Read the model definition and answer for the solid it produces. Units are mm, in the model's axes. A direction names the side the tool comes from. Coordinates: 2 decimals unless noted, no trailing zeros. Loops run counter-clockwise (first coordinate to the right, second up) from the corner with the lowest first, then second, coordinate; pieces in that order, holes last. Notation, with made-up numbers: (55, -6.5) -> (102, -6.5) arc R19 ccw to (102, 0.5) -> close; hole circle Ø8 at (48.25, 13.25). An arc over 180 degrees is marked (long way). Answer as CSV lines item,"result".
Autodesk Inventor part; units mm, degrees
ref_plane "YZ Plane" through (0, 0, 0) normal (1, 0, 0) x (0, 1, 0)
ref_plane "XZ Plane" through (0, 0, 0) normal (0, 1, 0) x (-1, 0, 0)
ref_plane "XY Plane" through (0, 0, 0) normal (0, 0, 1) x (1, 0, 0)
sketch "Sketch1" plane through (0, 0, 0) normal (0, 0, 1) x (1, 0, 0)
  line L0 (0, 0) -> (35, 0)
  line L1 (35, 0) -> (35, -31.5)
  line L2 (35, -31.5) -> (0, -31.5)
  line L3 (0, -31.5) -> (0, 0)
  dimension "d0" = 31.5
  dimension "d1" = 35
extrude "Extrusion1" add sketch "Sketch1" against normal blind 2.8
sketch "Sketch2" plane through (0, 0, 0) normal (0, 0, 1) x (1, 0, 0)
  line L0 (35, -31.5) -> (0, -31.5)
  line L1 (5.75, -37.2591) -> (29.25, -37.2591)
  line L2 (29.25, -37.2591) -> (29.25, -19.5)
  line L3 (29.25, -19.5) -> (5.75, -19.5)
  line L4 (5.75, -19.5) -> (5.75, -37.2591)
  point P0 (17.5, -19.5)
  point P1 (17.5, -31.5)
  dimension "d4" = 12
  dimension "d5" = 23.5
extrude "Extrusion2" cut sketch "Sketch2" against normal through all
sketch "Sketch3" plane through (0, 0, 0) normal (0, 0, 1) x (1, 0, 0)
  line L0 (0, 0) -> (35, 0)
  line L1 (0, -31.5) -> (0, 0)
  point P0 (8, -2.4)
  point P1 (27, -2.4)
  dimension "d8" = 8
  dimension "d9" = 19
  dimension "d10" = 2.4
hole "Hole1" at (8, -2.4, 0) at (27, -2.4, 0) direction (0, 0, -1) diameter 2.2 end through all
sketch "Sketch4" plane through (0, 0, 0) normal (0, 0, 1) x (1, 0, 0)
  line L0 (29.25, -19.5) -> (29.25, -31.5)
  line L1 (5.75, -31.5) -> (0, -31.5)
  line L2 (5.75, -31.5) -> (5.75, -19.5)
  point P0 (2.875, -25.5)
  point P1 (31.875, -25.5)
  point P2 (5.75, -25.5)
  point P3 (29.25, -25.5)
  point P4 (2.875, -31.5)
hole "Hole2" at (2.875, -25.5, 0) at (31.875, -25.5, 0) direction (0, 0, -1) diameter 1.567 end through all
properties part number "Servo Mount1"
Q1. A cutting plane is placed at C-C, the plane y = -2.4. Write down the section's boundary in (x, z).
Results:
outline,"(0, -2.8) -> (6.9, -2.8) -> (6.9, 0) -> (0, 0) -> close; (9.1, -2.8) -> (25.9, -2.8) -> (25.9, 0) -> (9.1, 0) -> close; (28.1, -2.8) -> (35, -2.8) -> (35, 0) -> (28.1, 0) -> close"
Q2. Find the intervals of material crossed by probe 1 along X at (y, z) = (-25.5, -1.4); probe 2 along X at (y, z) = (-2.4, -1.75); probe 3 along X at (y, z) = (-27, -0.75), in increasing order. Write a range as [from, to].
Results:
probe 1,"x = [0, 2.09], [3.66, 5.75], [29.25, 31.09], [32.66, 35]"
probe 2,"x = [0, 6.9], [9.1, 25.9], [28.1, 35]"
probe 3,"x = [0, 5.75], [29.25, 35]"
Q3. A cutting plane is placed at A-A, the plane y = -25.5. Write down the section's boundary in (x, z).
Results:
outline,"(0, -2.8) -> (2.09, -2.8) -> (2.09, 0) -> (0, 0) -> close; (3.66, -2.8) -> (5.75, -2.8) -> (5.75, 0) -> (3.66, 0) -> close; (29.25, -2.8) -> (31.09, -2.8) -> (31.09, 0) -> (29.25, 0) -> close; (32.66, -2.8) -> (35, -2.8) -> (35, 0) -> (32.66, 0) -> close"
Q4. For faces 1 (the face through (3.352, -24.878, -1.42)), 2 (the face through (29.25, -26, -1)), determine the directions among +Z, -Z, +X, -X, +Y, -Y from which every point of the face is accessible in a straight line to the end or side of a thin tool.
Results:
face 1,"+Z, -Z"
face 2,"+Z, -Z, -Y"
Q5. A cutting plane is placed at B-B, the plane x = 8. Write down the section's boundary in (y, z), and give its area (3 significant figures).
Results:
outline,"(-19.5, -2.8) -> (-3.5, -2.8) -> (-3.5, 0) -> (-19.5, 0) -> close; (-1.3, -2.8) -> (0, -2.8) -> (0, 0) -> (-1.3, 0) -> close"
area,"48.4 mm²"
Q6. Given pin 1 Ø1.4 at (x, z) = (15.5, -1.5) entering from -Y, flat-ended and moving along its own axis, determine where the tip first touches the part or whether it passes through.
Results:
pin 1,"stops at y = -19.5"
Q7. A cutting plane is placed at D-D, the plane z = -2.35. Give the number of separate pieces and of enclosed holes in the cut face, and give its area (3 significant figures).
Results:
separate pieces,"1"
enclosed holes,"4"
area,"809 mm²"
Q8. For a pull along Y with two mould halves and no side action, classify faces 3 (the face through (32, -31.5, -1)), 4 (the face through (17, 0, -1)), 5 (the face through (28.074, -2.162, -1.42)) as pulls with the +Y half, pulls with the -Y half, needs draft (parallel to the pull), parting line crosses it, or undercut.
Results:
face 3,"pulls with the -Y half"
face 4,"pulls with the +Y half"
face 5,"undercut"
